from build123d import *

# Parameters (mm, degrees)
BOSS_EXTRUDE2_DEPTH = 2
SKETCH2_R           = 2.15
CUT_EXTRUDE1_DEPTH  = 10
CUT_EXTRUDE3_DEPTH  = 30
BOSS_EXTRUDE4_DEPTH = 2
SKETCH9_W           = 20
SKETCH9_H           = 40
BOSS_EXTRUDE5_DEPTH = 2
CUT_EXTRUDE4_DEPTH  = 2
BOSS_EXTRUDE6_DEPTH = 2
BOSS_EXTRUDE7_DEPTH = 2
CUT_EXTRUDE5_DEPTH  = 2


with BuildPart() as part:
    # Sketch1 → Boss-Extrude2 (new body)
    with BuildSketch(Plane(origin=(0, 0, 0), x_dir=(1, 0, 0), z_dir=(0, 1, 0))):
        Polygon((102.5, 0), (51.25, 88.767603888), (-51.25, 88.767603888), (-102.5, 0), (-51.25, -88.767603888), (51.25, -88.767603888), align=None)
        Polygon((73.632486541, 0), (36.81624327, 63.767603888), (10, 63.767603888), (10, 45.767603888), (30, 45.767603888), (30, -45.767603888), (10, -45.767603888), (10, -63.767603888), (36.81624327, -63.767603888), align=None, mode=Mode.SUBTRACT)
        Polygon((-10, 63.767603888), (-36.81624327, 63.767603888), (-73.632486541, 0), (-36.81624327, -63.767603888), (-10, -63.767603888), (-10, -45.767603888), (-30, -45.767603888), (-30, 45.767603888), (-10, 45.767603888), align=None, mode=Mode.SUBTRACT)
    extrude(amount=BOSS_EXTRUDE2_DEPTH)

    # Sketch2 → Cut-Extrude1 (cut)
    with BuildSketch(Plane(origin=(0, 2, 0), x_dir=(1, 0, 0), z_dir=(0, 1, 0))):
        with Locations((-72.544872981, -41.883801944)):
            Circle(SKETCH2_R)
        with Locations((-63.884618943, -36.883801944)):
            Circle(SKETCH2_R)
        with Locations((-72.544872981, 41.883801944)):
            Circle(SKETCH2_R)
        with Locations((-63.884618943, 36.883801944)):
            Circle(SKETCH2_R)
        with Locations((0, 83.767603888)):
            Circle(SKETCH2_R)
        with Locations((0, 73.767603888)):
            Circle(SKETCH2_R)
        with Locations((72.544872981, 41.883801944)):
            Circle(SKETCH2_R)
        with Locations((63.884618943, 36.883801944)):
            Circle(SKETCH2_R)
        with Locations((72.544872981, -41.883801944)):
            Circle(SKETCH2_R)
        with Locations((63.884618943, -36.883801944)):
            Circle(SKETCH2_R)
        with Locations((0, -83.767603888)):
            Circle(SKETCH2_R)
        with Locations((0, -73.767603888)):
            Circle(SKETCH2_R)
    extrude(amount=-CUT_EXTRUDE1_DEPTH, mode=Mode.SUBTRACT)

    # Sketch7 → Cut-Extrude3 (cut)
    with BuildSketch(Plane.XZ):
        Polygon((73.632486541, 0), (36.81624327, 63.767603888), (-36.81624327, 63.767603888), (-73.632486541, 0), (-36.81624327, -63.767603888), (36.81624327, -63.767603888), align=None)
    extrude(amount=-CUT_EXTRUDE3_DEPTH, mode=Mode.SUBTRACT)



with BuildPart() as body_2:
    # Sketch8 → Boss-Extrude4 (new body)
    with BuildSketch(Plane.XZ):
        Polygon((2.980762114, 54.837168574), (-23, 39.837168574), (0, 0), (25.980762114, 15), align=None)
        Polygon((-23, 39.837168574), (-48.980762114, 24.837168574), (-2.980762114, -54.837168574), (48.980762114, -24.837168574), (25.980762114, 15), (0, 0), align=None)
    extrude(amount=-BOSS_EXTRUDE4_DEPTH)


with BuildPart() as part_1:
    add(part.part)

    add(body_2.part)  # Boss-Extrude5 merges body 2
    # Sketch9 → Boss-Extrude5 (add)
    with BuildSketch(Plane(origin=(0, 0, 0), x_dir=(-1, 0, 0), z_dir=(0, -1, 0))):
        Polygon((60.224364905, -23.223547906), (25.583348754, -3.223547906), (15.583348754, -20.544055982), (50.224364905, -40.544055982), align=None)
        with Locations((0, -43.767603888)):
            Rectangle(SKETCH9_W, SKETCH9_H)
        Polygon((-60.224364905, -23.223547906), (-25.583348754, -3.223547906), (-15.583348754, -20.544055982), (-50.224364905, -40.544055982), align=None)
        Polygon((-50.224364905, 40.544055982), (-15.583348754, 20.544055982), (-25.583348754, 3.223547906), (-60.224364905, 23.223547906), align=None)
        with Locations((0, 43.767603888)):
            Rectangle(SKETCH9_W, SKETCH9_H)
        Polygon((60.224364905, 23.223547906), (25.583348754, 3.223547906), (15.583348754, 20.544055982), (50.224364905, 40.544055982), align=None)
    extrude(amount=-BOSS_EXTRUDE5_DEPTH)

    # Sketch10 → Cut-Extrude4 (cut)
    with BuildSketch(Plane(origin=(0, 0, 0), x_dir=(-1, 0, 0), z_dir=(0, -1, 0))):
        Polygon((60.224364905, -23.223547906), (98.115262944, -45.099868089), (121.783609118, 0), (103.941012458, 48.463366139), (60.224364905, 23.223547906), align=None)
        Polygon((10, -107.520244253), (60.891804559, -105.467699261), (93.941012458, -65.783874214), (50.224364905, -40.544055982), (10, -63.767603888), align=None)
        Polygon((-88.115262944, -62.420376164), (-60.891804559, -105.467699261), (-10, -114.247240353), (-10, -63.767603888), (-50.224364905, -40.544055982), align=None)
        Polygon((-98.115262944, 45.099868089), (-121.783609118, 0), (-103.941012458, -48.463366139), (-60.224364905, -23.223547906), (-60.224364905, 23.223547906), align=None)
        Polygon((-10, 107.520244253), (-60.891804559, 105.467699261), (-93.941012458, 65.783874214), (-50.224364905, 40.544055982), (-10, 63.767603888), align=None)
        Polygon((88.115262944, 62.420376164), (60.891804559, 105.467699261), (10, 114.247240353), (10, 63.767603888), (50.224364905, 40.544055982), align=None)
    extrude(amount=-CUT_EXTRUDE4_DEPTH, mode=Mode.SUBTRACT)

    # Sketch12 → Boss-Extrude6 (add)
    with BuildSketch(Plane.XZ):
        Polygon((-81.205127019, -46.883801944), (-86.205127019, -38.223547906), (-81.875, -35.723547906), (-71.875, -53.044055982), (-76.205127019, -55.544055982), align=None)
        Polygon((-81.205127019, 46.883801944), (-86.205127019, 38.223547906), (-81.875, 35.723547906), (-71.875, 53.044055982), (-76.205127019, 55.544055982), align=None)
        Polygon((0, 93.767603888), (-10, 93.767603888), (-10, 88.767603888), (10, 88.767603888), (10, 93.767603888), align=None)
        Polygon((81.205127019, 46.883801944), (76.205127019, 55.544055982), (71.875, 53.044055982), (81.875, 35.723547906), (86.205127019, 38.223547906), align=None)
        Polygon((81.205127019, -46.883801944), (86.205127019, -38.223547906), (81.875, -35.723547906), (71.875, -53.044055982), (76.205127019, -55.544055982), align=None)
        Polygon((0, -93.767603888), (10, -93.767603888), (10, -88.767603888), (-10, -88.767603888), (-10, -93.767603888), align=None)
    extrude(amount=-BOSS_EXTRUDE6_DEPTH)

    # Sketch14 → Boss-Extrude7 (add)
    with BuildSketch(Plane(origin=(0, 2, 0), x_dir=(1, 0, 0), z_dir=(0, 1, 0))):
        Polygon((-18.239092363, 54.408965344), (-26.239092363, 40.552558883), (-14.980762114, 34.052558883), (-10, 42.679491924), (-10, 49.65212315), align=None)
        Polygon((41.961524227, 12.679491924), (36.980762114, 4.052558883), (48.239092363, -2.447441117), (56.239092363, 11.408965344), (48, 16.165807537), align=None)
        Polygon((26.239092363, -40.552558883), (14.980762114, -34.052558883), (10, -42.679491924), (10, -49.65212315), (18.239092363, -54.408965344), align=None)
        Polygon((-36.980762114, -4.052558883), (-48.239092363, 2.447441117), (-56.239092363, -11.408965344), (-48, -16.165807537), (-41.961524227, -12.679491924), align=None)
    extrude(amount=-BOSS_EXTRUDE7_DEPTH)

    # Sketch15 → Cut-Extrude5 (cut)
    with BuildSketch(Plane(origin=(0, 2, 0), x_dir=(1, 0, 0), z_dir=(0, 1, 0))):
        Polygon((-18.239092363, 54.408965344), (-14.774990748, 52.408965344), (-22.774990748, 38.552558883), (-26.239092363, 40.552558883), align=None)
        Polygon((-44.774990748, 0.447441117), (-48.239092363, 2.447441117), (-56.239092363, -11.408965344), (-52.774990748, -13.408965344), align=None)
        Polygon((18.239092363, -54.408965344), (14.774990748, -52.408965344), (22.774990748, -38.552558883), (26.239092363, -40.552558883), align=None)
        Polygon((44.774990748, -0.447441117), (48.239092363, -2.447441117), (56.239092363, 11.408965344), (52.774990748, 13.408965344), align=None)
    extrude(amount=-CUT_EXTRUDE5_DEPTH, mode=Mode.SUBTRACT)


solid = part_1.part
Could you check a few things on this model? Use its own coordinates, in mm. A direction names the side the tool comes from. Give positions to 0.01 mm unless a question says otherwise; leave off trailing zeros. Loops run counter-clockwise (first coordinate to the right, second up) from the corner with the lowest first, then second, coordinate; pieces in that order, holes last. Notation, with made-up numbers: (51.25, 8) -> (56.25, 8) arc R17 ccw to (56.25, 28) -> close; hole circle Ø9 at (-9.5, 8.5). An arc over 180 degrees is marked (long way). Return JSON: item names as keys, results as strings.
Item 1: If we section it at C-C on y = 1.2: Count the separate pieces of the cut face and the enclosed holes in it, plus the area to 3 significant figures.
Geometry results:
{"separate pieces": "1", "enclosed holes": "12", "area": "11,900 mm²"}
Item 2: If we section it at B-B on z = 29: List the corners of the cut face in (x, y) for me.
Geometry results:
{"outline": "(-70.23, 0) -> (17.9, 0) -> (17.9, 2) -> (-70.23, 2) -> close; (30.23, 0) -> (70.23, 0) -> (70.23, 2) -> (30.23, 2) -> close"}
Item 3: If we section it at D-D on z = -68: List the corners of the cut face in (x, y) for me, plus the area to 3 significant figures.
Geometry results:
{"outline": "(-10, 0) -> (10, 0) -> (10, 2) -> (-10, 2) -> close", "area": "40.0 mm²"}
Item 4: Which directions (+Z, -Z, +X, -X, +Y, -Y) give clear straight access to the entire face, cutting with the end or side of a thin tool? Please do faces 4 (the flat face through (18.932, 1.014, 36.334)), 5 (the flat face through (-22.82, 0.99, 39.94)), 6 (the flat face through (-48.83, 1.01, 6.58)).
Geometry results:
{"face 4": "+Y, -Y", "face 5": "+Z, +Y, -Y", "face 6": "-X, +Y, -Y"}
Item 5: We'd pull the mould along Z, two halves only. Please class faces 1 (the flat face through (-81.275, 0.986, -46.763)), 2 (the flat face through (-40.823, 1.014, 1.834)), 3 (the flat face through (18.72, 1.01, 45.58)): +Z half, -Z half, draft (parallel to the pull), parting line (faces both ways), or undercut.
Geometry results:
{"face 1": "-Z half", "face 2": "undercut", "face 3": "+Z half"}
Item 6: If we section it at A-A on x = 0: List the corners of the cut face in (y, z) for me.
Geometry results:
{"outline": "(0, -93.77) -> (2, -93.77) -> (2, -85.92) -> (0, -85.92) -> close; (0, -81.62) -> (2, -81.62) -> (2, -75.92) -> (0, -75.92) -> close; (0, -71.62) -> (2, -71.62) -> (2, 71.62) -> (0, 71.62) -> close; (0, 75.92) -> (2, 75.92) -> (2, 81.62) -> (0, 81.62) -> close; (0, 85.92) -> (2, 85.92) -> (2, 93.77) -> (0, 93.77) -> close"}
Item 7: I need wall thicknesses on L1, parallel to Z at x = 0, y = 0.6; L2, parallel to X at y = 1.3, z = 35; L3, parallel to X at y = 1.95, z = -60.5. Which ranges of each line are inside material? Lowest first, please. Write a range as from..to.
Geometry results:
{"L1": "z = -93.77..-85.92, -81.62..-75.92, -71.62..71.62, 75.92..81.62, 85.92..93.77", "L2": "x = -80.62..-64.92, -62.85..-40.62, -31.38..16.62, 40.62..62.85, 64.92..80.62", "L3": "x = -10..10"}
Item 8: I'm going to push flat-ended pins straight in: pin 1 (4 mm diameter, centred on x = 63.88, z = -36.88, fed in from +Y); pin 2 (0.6 mm diameter, centred on y = 1, z = 76.5, fed in from +X); pin 3 (0.6 mm diameter, centred on y = 0.5, z = 80, fed in from -X). Where does each tip first touch, or does it pass through?
Geometry results:
{"pin 1": "passes through", "pin 2": "stops at x = 10", "pin 3": "stops at x = -10"}
